Geometry: final body of the model. Coordinates: model frame, mm. A direction names the side the tool comes from. Give positions to 0.01 mm unless a question says otherwise; leave off trailing zeros. Loops run counter-clockwise (first coordinate to the right, second up) from the corner with the lowest first, then second, coordinate; pieces in that order, holes last.
from build123d import *

# Parameters (mm, degrees)
F0_W     = 10
F0_H     = 10
F0_W_2   = 22.3
F0_H_2   = 32.3
F0_H_3   = 32.8545699317
F1_DEPTH = 7
F2_D     = 3.3


with BuildPart() as f1:
    # F0 (on Top) → F1 (new body)
    with BuildSketch(Plane.XY):
        with Locations((-15.4388597772, 17.3551567454)):
            Rectangle(F0_W, F0_H)
        with Locations((0.7111402228, 17.3551567454)):
            Rectangle(F0_W_2, F0_H)
        with Locations((-15.4388597772, -3.7948432546)):
            Rectangle(F0_W, F0_H_2)
        with Locations((16.8611402228, 17.3551567454)):
            Rectangle(F0_W, F0_H)
        with Locations((16.8611402228, -4.0721282204)):
            Rectangle(F0_W, F0_H_3)
    extrude(amount=F1_DEPTH)

    # F2 (through all)
    with Locations(Plane(origin=(0, 0, 0), x_dir=(1, 0, 0), z_dir=(0, 0, -1))):
        with Locations((-14.7888597772, -16.7051567454), (16.2111402228, -16.7051567454), (-14.7888597772, 14.8494131863), (16.2111402228, 14.8494131863)):
            Hole(F2_D / 2)


solid = f1.part
Item 1: Ray query, probe 1 along X at (y, z) = (-11, 5.75); probe 2 along Y at (x, z) = (-16, 1.25); probe 3 along X at (y, z) = (17, 3.75). Return the intervals inside material, ascending.
Values follow:
probe 1: x = -20.44 to -10.44, 11.86 to 21.86
probe 2: y = -19.94 to -15.97, -13.73 to 15.58, 17.83 to 22.36
probe 3: x = -20.44 to -16.41, -13.17 to 14.59, 17.83 to 21.86
Item 2: Draft query along Y for faces 4 (the face through (-10.439, -4, 3)), 5 (the face through (-15.55, -13.386, 3.549)), 6 (the face through (1, 12.355, 3)), 7 (the face through (16.43, 15.07, 3.55)). Return one class per face: +Y half, -Y half, draft (parallel to the pull), parting line (faces both ways), or undercut.
Values follow:
face 4: draft
face 5: undercut
face 6: -Y half
face 7: undercut
Item 3: Pin query (flat end, axial travel): pin 1 (3.5 mm diameter, centred on x = -15.5, z = 3.5, fed in from -Y); pin 2 (3.5 mm diameter, centred on x = 4.5, z = 3, fed in from -Y); pin 3 (10 mm diameter, centred on x = 6, y = -7, fed in from -Z). Return the tip coordinate at first contact, or that it passes through.
Values follow:
pin 1: stops at y = -19.94
pin 2: stops at y = 12.36
pin 3: passes through
Item 4: Section query A-A on y = -6. Return loops of the section in (x, z), plus the area to 3 significant figures.
Values follow:
outline: (-20.44, 0) - (-10.44, 0) - (-10.44, 7) - (-20.44, 7) - close; (11.86, 0) - (21.86, 0) - (21.86, 7) - (11.86, 7) - close
area: 140 mm2
Item 5: Section query C-C on x = -5. Return loops of the section in (y, z), plus the area to 3 significant figures.
Values follow:
outline: (12.36, 0) - (22.36, 0) - (22.36, 7) - (12.36, 7) - close
area: 70.0 mm2
Item 6: Section query B-B on z = 2. Return loops of the section in (x, y).
Values follow:
outline: (-20.44, -19.94) - (-10.44, -19.94) - (-10.44, 12.36) - (11.86, 12.36) - (11.86, -20.5) - (21.86, -20.5) - (21.86, 22.36) - (-20.44, 22.36) - close; hole circle Ø3.3 at (-14.79, -14.85); hole circle Ø3.3 at (-14.79, 16.71); hole circle Ø3.3 at (16.21, -14.85); hole circle Ø3.3 at (16.21, 16.71)
Item 7: Set-up query: faces 1 (the face through (11.861, -4, 3)), 2 (the face through (0, 16, 0)), 3 (the face through (-16, -19.945, 3)). Return all of +Z, -Z, +X, -X, +Y, -Y with unobstructed straight access to the full face (end or side cutting, diameter ignored); none if empty.
Values follow:
face 1: +Z, -Z, -Y
face 2: -Z, +X, -X, +Y, -Y
face 3: +Z, -Z, -X, -Y
